The listing builds one solid part. Answer for the finished solid, in the listing's coordinates (mm). A direction names the side the tool comes from. Round coordinates to 2 decimals unless told otherwise and drop trailing zeros. Loops run counter-clockwise (first coordinate to the right, second up) from the corner with the lowest first, then second, coordinate; pieces in that order, holes last. Notation, with made-up numbers: (-36, 6) -> (-22, 6) arc R22 ccw to (-22, 36) -> close; hole circle Ø4 at (48.5, 24). An arc over 180 degrees is marked (long way). Use a Markdown table: item, result. Add a question column.
Q1. Section B-B on z = -14.5 is taken. Give the vertices of the cut face in (x, y).
Q2. Section A-A on y = -3.5 is taken. Give the vertices of the cut face in (x, z).
Q3. Consider line 1 (X direction, y = -3, z = -9.25); line 2 (X direction, y = -2.75, z = -46); line 3 (X direction, y = 0.65, z = -27.5). Determine where each line is inside the solid, lowest interval first.
Q4. Section D-D on z = -45.75 is taken. Give the vertices of the cut face in (x, y), then the cut area to 3 significant figures.
Q5. Which of the six approach directions +Z, -Z, +X, -X, +Y, -Y give full straight-line access (tool end or side, diameter ignored) to faces 5 (the flat face through (64, -8, -9)), 6 (the cylindrical face through (15.82, -3.94, -44.25))?
Q6. Section C-C on x = 13 is taken. Give the vertices of the cut face in (y, z).
Q7. For a pull along X with two mould halves and no side action, classify faces 1 (the cylindrical face through (65.237, -3.944, -9.055)), 2 (the flat face through (16, -8, -46)), 3 (the flat face through (25.5, -4, -28)), 4 (the flat face through (6, -4, -28)) as released by +X, released by -X, zero draft, split by the parting line, or undercut.
Q8. Given pin 1 Ø2.5 at (y, z) = (-5.5, -27) entering from -X; pin 2 Ø1.5 at (y, z) = (-4.5, -28.5) entering from +X; pin 3 Ø21 at (x, z) = (76.6, -27.5) entering from -Y, each flat-ended and moving along its own axis, determine where each tip first touches the part or whether it passes through.
from build123d import *

# Parameters (mm, degrees)
SKETCH1_W           = 90
SKETCH1_H           = 55
BOSS_EXTRUDE1_DEPTH = 1
SKETCH2_R           = 6.6
SKETCH2_W           = 19.5
SKETCH2_H           = 12.75
CUT_EXTRUDE1_DEPTH  = 106.479855897
SKETCH3_R           = 1.5
SKETCH3_R_2         = 0.194235627
SKETCH3_W           = 19.5
SKETCH3_H           = 5
BOSS_EXTRUDE4_DEPTH = 8


with BuildPart() as part:
    # Sketch1 → Boss-Extrude1 (new body)
    with BuildSketch(Plane(origin=(0, 0, 0), x_dir=(1, 0, 0), z_dir=(0, 1, 0))):
        with Locations((45, 27.5)):
            Rectangle(SKETCH1_W, SKETCH1_H)
    extrude(amount=BOSS_EXTRUDE1_DEPTH)

    # Sketch2 → Cut-Extrude1 (cut, through all)
    with BuildSketch(Plane(origin=(0, 1, 0), x_dir=(1, 0, 0), z_dir=(0, 1, 0))):
        with Locations(Location((76.6, 27.5, 0), (0, 0, 270))):
            Circle(SKETCH2_R)
        with Locations((15.75, 36.375)):
            Rectangle(SKETCH2_W, SKETCH2_H)
        with Locations((15.75, 18.625)):
            Rectangle(SKETCH2_W, SKETCH2_H)
    extrude(amount=-CUT_EXTRUDE1_DEPTH, mode=Mode.SUBTRACT)

    # Sketch3 → Boss-Extrude4 (add)
    # profile 1 of 7: a face of its own
    with BuildSketch(Plane.XZ):
        with Locations(Location((15.75, -9.25, 0), (0, 0, 270))):
            Circle(SKETCH3_R)
        with Locations(Location((15.75, -9.25, 0), (0, 0, 270))):
            Circle(SKETCH3_R_2, mode=Mode.SUBTRACT)
    # profile 2 of 7: a face of its own
    with BuildSketch(Plane.XZ):
        with Locations(Location((15.75, -45.75, 0), (0, 0, 270))):
            Circle(SKETCH3_R)
    # profile 3 of 7: a face of its own
    with BuildSketch(Plane.XZ):
        with Locations(Location((63.75, -9.25, 0), (0, 0, 270))):
            Circle(SKETCH3_R)
    # profile 4 of 7: a face of its own
    with BuildSketch(Plane.XZ):
        with Locations(Location((63.75, -45.75, 0), (0, 0, 270))):
            Circle(SKETCH3_R)
    # profile 5 of 7: a face of its own
    with BuildSketch(Plane.XZ):
        with Locations(Location((63.75, -27.411126752, 0), (0, 0, 270))):
            Circle(SKETCH3_R)
    # profile 6 of 7: a face of its own
    with BuildSketch(Plane.XZ):
        with Locations(Location((42.289365933, -27.411126752, 0), (0, 0, 270))):
            Circle(SKETCH3_R)
    # profile 7 of 7: a face of its own
    with BuildSketch(Plane.XZ):
        with Locations((15.75, -27.5)):
            Rectangle(SKETCH3_W, SKETCH3_H)
    extrude(amount=BOSS_EXTRUDE4_DEPTH)


solid = part.part
Checked values:
| question | item | result |
|---|---|---|
| 1 | outline | (0, 0) -> (6, 0) -> (6, 1) -> (0, 1) -> close; (25.5, 0) -> (90, 0) -> (90, 1) -> (25.5, 1) -> close |
| 2 | outline | (6, -30) -> (25.5, -30) -> (25.5, -25) -> (6, -25) -> close; circle Ø3 at (15.75, -45.75); circle Ø3 at (15.75, -9.25); circle Ø3 at (42.29, -27.41); circle Ø3 at (63.75, -45.75); circle Ø3 at (63.75, -27.41); circle Ø3 at (63.75, -9.25); hole circle Ø0.39 at (15.75, -9.25) |
| 3 | line 1 | x = 14.25 to 15.56, 15.94 to 17.25, 62.25 to 65.25 |
| 3 | line 2 | x = 14.27 to 17.23, 62.27 to 65.23 |
| 3 | line 3 | x = 0 to 70, 83.2 to 90 |
| 4 | outline | (0, 0) -> (14.25, 0) -> (14.25, -8) -> (17.25, -8) -> (17.25, 0) -> (62.25, 0) -> (62.25, -8) -> (65.25, -8) -> (65.25, 0) -> (90, 0) -> (90, 1) -> (0, 1) -> close |
| 4 | area | 138 mm2 |
| 5 | face 5 | +Z, -Z, +X, -X, -Y |
| 5 | face 6 | -Y |
| 6 | outline | (-8, -30) -> (1, -30) -> (1, -25) -> (-8, -25) -> close; (0, -55) -> (1, -55) -> (1, -42.75) -> (0, -42.75) -> close; (0, -12.25) -> (1, -12.25) -> (1, 0) -> (0, 0) -> close |
| 7 | face 1 | undercut |
| 7 | face 2 | zero draft |
| 7 | face 3 | undercut |
| 7 | face 4 | released by -X |
| 8 | pin 1 | stops at x = 6 |
| 8 | pin 2 | stops at x = 65.21 |
| 8 | pin 3 | stops at y = 0 |
